Model file for the job. Use its own axes, mm. A direction names the side the tool comes from. Give positions to 0.01 mm unless a question says otherwise; leave off trailing zeros. Order: outer loops, then holes, each group sorted by start corner. A loop starts at its lowest first (then second) coordinate and runs counter-clockwise, first axis right, second up. Notation, with made-up numbers: (14.5, -32.5) -> (40.5, -32.5) arc R15 cw to (40.5, -15.5) -> close; hole circle Ø9 at (79, 78.5). An arc over 180 degrees is marked (long way). Use CSV: the item, a comma, the result in double quotes. Start each with the question number.
1. Cut at B-B on z = 5.35. List the corners of the cut face in (x, y).
2. Cut at A-A on x = 11. List the corners of the cut face in (y, z).
3. Wall check: line 1 (Z direction, x = 11, y = -26.25); line 2 (Y direction, x = 12, z = 12); line 3 (Y direction, x = 20.5, z = 40). Give the ranges that are in metal, low to high. Write a range as from..to.
4. Cut at D-D on x = 46. List the corners of the cut face in (y, z), then the cut area to 3 significant figures.
5. Pull direction X, two halves, no side cores. Call faces 6 (the flat face through (52, 12, 21)), 7 (the cylindrical face through (12.19, -26.12, 35.74)), 8 (the flat face through (4.7, -0.7, 42)): released by +X, released by -X, zero draft, split by the parting line, or undercut.
6. Drop flat-ended pins along their axis: pin 1 (21 mm diameter, centred on x = 39.5, z = 30.5, fed in from -Y); pin 2 (6 mm diameter, centred on y = 4.5, z = 34, fed in from +X); pin 3 (4 mm diameter, centred on y = -25, z = 25.5, fed in from +X). Give the stop position or say it passes through.
7. 3-axis set-ups, long thin cutter, end or side, ignore diameter. For faces 1 (the flat face through (5, -7, 21)), 2 (the flat face through (14.2, -26, 21)), 3 (the cylindrical face through (12.5, -26.1, 5.4)), 4 (the flat face through (7, -28.651, 21)), 5 (the flat face through (4.7, -0.7, 0)): which of +Z, -Z, +X, -X, +Y, -Y reach the whole face in a straight line?
8. Cut at C-C on z = 30. List the corners of the cut face in (x, y), then the cut area to 3 significant figures.
```python
from build123d import *

# Parameters (mm, degrees)
F0_W     = 9.2
F0_H     = 5
F1_DEPTH = 42
F3_D     = 3
F3_DEPTH = 12
F4_D     = 3
F4_DEPTH = 12


with BuildPart() as f1:
    # F0 (on Top) → F1 (new body)
    with BuildSketch(Plane.XY):
        Polygon((0, 14.349465), (0, 9.349465), (5, 9.349465), (52, 9.349465), (52, 14.349465), align=None)
        Polygon((5, 9.349465), (0, 9.349465), (0, -28.650535), (5, -28.650535), (5, -23.650535), align=None)
        with Locations((9.6, -26.150535)):
            Rectangle(F0_W, F0_H)
    extrude(amount=F1_DEPTH)

    # F3
    with Locations(Plane.XZ.offset(28.650535)):
        with Locations((11, 36.65)):
            Hole(F3_D / 2, depth=F3_DEPTH)

    # F4
    with Locations(Plane.XZ.offset(28.650535)):
        with Locations((11, 5.35)):
            Hole(F4_D / 2, depth=F4_DEPTH)


solid = f1.part
```
Verdict:
1,outline,"(0, -28.65) -> (9.5, -28.65) -> (9.5, -23.65) -> (5, -23.65) -> (5, 9.35) -> (52, 9.35) -> (52, 14.35) -> (0, 14.35) -> close; (12.5, -28.65) -> (14.2, -28.65) -> (14.2, -23.65) -> (12.5, -23.65) -> close"
2,outline,"(-28.65, 0) -> (-23.65, 0) -> (-23.65, 3.85) -> (-28.65, 3.85) -> close; (-28.65, 6.85) -> (-23.65, 6.85) -> (-23.65, 35.15) -> (-28.65, 35.15) -> close; (-28.65, 38.15) -> (-23.65, 38.15) -> (-23.65, 42) -> (-28.65, 42) -> close; (9.35, 0) -> (14.35, 0) -> (14.35, 42) -> (9.35, 42) -> close"
3,line 1,"0..3.85, 6.85..35.15, 38.15..42"
3,line 2,"-28.65..-23.65, 9.35..14.35"
3,line 3,"9.35..14.35"
4,outline,"(9.35, 0) -> (14.35, 0) -> (14.35, 42) -> (9.35, 42) -> close"
4,area,"210 mm^2"
5,face 6,"released by +X"
5,face 7,"undercut"
5,face 8,"zero draft"
6,pin 1,"y = 9.35"
6,pin 2,"x = 5"
6,pin 3,"x = 14.2"
7,face 1,"+Z, -Z, +X"
7,face 2,"+Z, -Z, +X, -Y"
7,face 3,"-Y"
7,face 4,"+Z, -Z, +X, -X, -Y"
7,face 5,"-Z, +X, -X, +Y, -Y"
8,outline,"(0, -28.65) -> (14.2, -28.65) -> (14.2, -23.65) -> (5, -23.65) -> (5, 9.35) -> (52, 9.35) -> (52, 14.35) -> (0, 14.35) -> close"
8,area,"496 mm^2"
